Geometry check sheet. Reference: drawing and pictorial views, mm from the part's lowest x, y, z. Give positions to 0.01 mm unless a question says otherwise; leave off trailing zeros. Write each loop counter-clockwise with the first axis right and the second up, starting at its lowest first coordinate (ties: lowest second). Pieces come first, ordered by that corner, then holes.
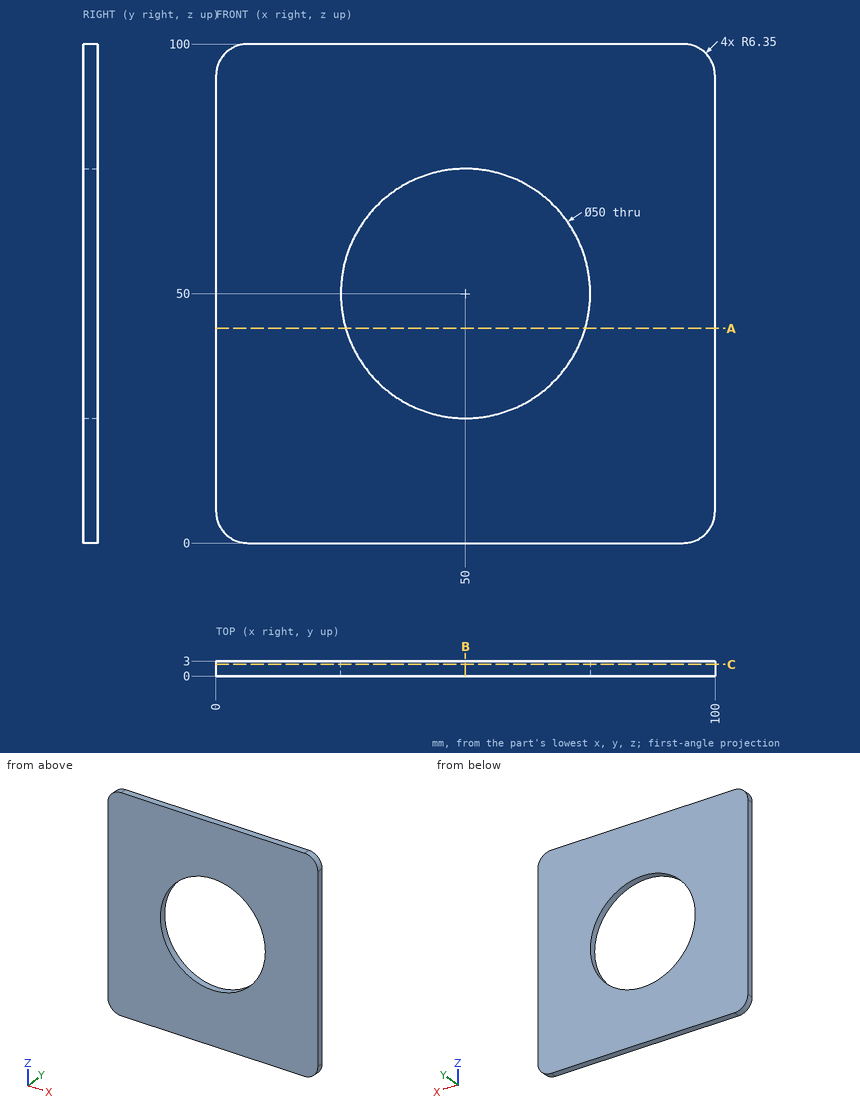
Item 1: Sectioned sample at C-C on y = 2.35. Record the cut outline in (x, z), then the cut area to 3 significant figures.
Answer key:
outline: (0, 6.35) arc R6.35 ccw to (6.35, 0) - (93.65, 0) arc R6.35 ccw to (100, 6.35) - (100, 93.65) arc R6.35 ccw to (93.65, 100) - (6.35, 100) arc R6.35 ccw to (0, 93.65) - close; hole circle Ø50 at (50, 50)
area: 8,000 mm2
Item 2: Sectioned sample at B-B on x = 50. Record the cut outline in (y, z), then the cut area to 3 significant figures.
Answer key:
outline: (0, 0) - (3, 0) - (3, 25) - (0, 25) - close; (0, 75) - (3, 75) - (3, 100) - (0, 100) - close
area: 150 mm2
Item 3: Depth check by flat-ended pin: pin 1 (1.5 mm diameter, centred on x = 48, y = 1, fed in from -Z). Enter the tip coordinate at first touch or a pass-through.
Answer key:
pin 1: stops at z = 0
Item 4: Sectioned sample at A-A on z = 43. Record the cut outline in (x, y).
Answer key:
outline: (0, 0) - (26, 0) - (26, 3) - (0, 3) - close; (74, 0) - (100, 0) - (100, 3) - (74, 3) - close
Item 5: Scan lines: line 1 along Z through (x, y) = (50, 2.15); line 2 along Z through (x, y) = (72.5, 1.55); line 3 along X through (y, z) = (1.5, 57). Record each from-to range of solid material in increasing order.
Answer key:
line 1: z = 0 to 25, 75 to 100
line 2: z = 0 to 39.1, 60.9 to 100
line 3: x = 0 to 26, 74 to 100
